Autodesk Inventor part; units mm, degrees
ref_plane "YZ Plane" through (0, 0, 0) normal (1, 0, 0) x (0, 1, 0)
ref_plane "XZ Plane" through (0, 0, 0) normal (0, 1, 0) x (-1, 0, 0)
ref_plane "XY Plane" through (0, 0, 0) normal (0, 0, 1) x (1, 0, 0)
sketch "Sketch1" plane through (0, 0, 0) normal (0, 0, 1) x (1, 0, 0)
  line L0 (0, 0) -> (177.8, 0)
  line L1 (177.8, 0) -> (177.8, 50.8)
  line L2 (177.8, 50.8) -> (0, 50.8)
  line L3 (0, 50.8) -> (0, 0)
  dimension "d0" = 177.8
  dimension "d1" = 50.8
extrude "Extrusion1" add sketch "Sketch1" along normal blind 25.4
shell "Shell1" thickness 1.5875 removed faces 2 at (0, 33.8667, 16.9333) at (177.8, 16.9333, 16.9333)
sketch "Sketch2" plane through (0, 0, 25.4) normal (0, 0, 1) x (1, 0, 0)
  line L0 (0, 0) -> (63.5, 0) construction
  line L1 (63.5, 0) -> (63.5, 25.4) construction
  line L2 (63.5, 25.4) -> (0, 25.4) construction
  line L3 (0, 25.4) -> (0, 0) construction
  dimension "d5" = 63.5
  dimension "d13" = 25.4
hole "Hole1" at (63.5, 25.4, 25.4) direction (0, 0, -1) diameter 28.575 end through all
hole "Hole2" at (12.7, 12.7, 25.4) direction (0, 0, -1) diameter 5.1594 end through all
hole "Hole3" at (38.1, 12.7, 25.4) direction (0, 0, -1) diameter 5.1594 end through all
hole "Hole4" at (165.1, 12.7, 25.4) direction (0, 0, -1) diameter 5.1594 end through all
hole "Hole5" at (139.7, 12.7, 25.4) direction (0, 0, -1) diameter 5.1594 end through all
hole "Hole6" at (12.7, 0, 12.7) direction (0, 1, 0) diameter 5.1594 depth 1.5875 tip angle 118
hole "Hole7" at (165.1, 0, 12.7) direction (0, 1, 0) diameter 5.1594 depth 3.175 tip angle 118
properties part number "1x2 5 in Beam Flywheel Mount"
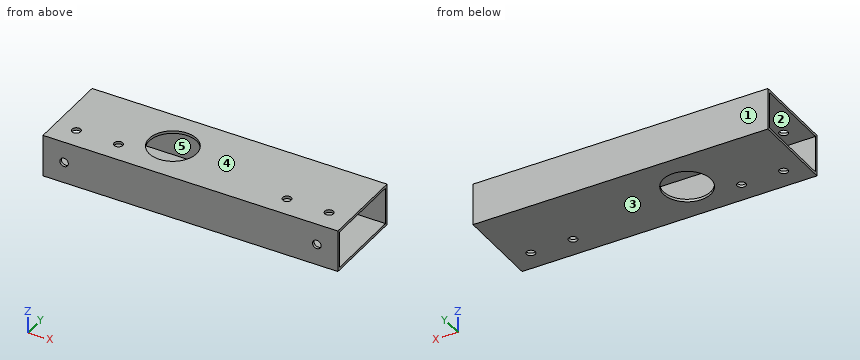
Design review of the part built by this model. Coordinates are the model's own, in mm. Face numbers are marked on the shaded views. A direction names the side the tool comes from. Round coordinates to 2 decimals unless told otherwise and drop trailing zeros. Write each loop counter-clockwise with the first axis right and the second up, starting at its lowest first coordinate (ties: lowest second). Pieces come first, ordered by that corner, then holes. Notation, with made-up numbers: (45, -18) - (97, -18) arc R11 ccw to (97, 2) - close; hole circle Ø4 at (1.25, 59). An arc over 180 degrees is marked (long way). Return JSON: item names as keys, results as strings. Group by question number.
Item 1: We need section A-A on z = 12.7. Write out the cut boundary in (x, y), and give its area (3 significant figures).
Item 2: For probe 1 along X at (y, z) = (0.6, 12.7); probe 2 along Z at (x, y) = (23.5, 4); probe 3 along Y at (x, z) = (165.1, 24.7), list the stretches that pass through material, from the lowest coordinate up. Write a range as [from, to].
Item 3: The part is to be moulded in two halves that separate along Y. For the marked faces 1, 2 and 3, say which applies: pulls with the +Y half, pulls with the -Y half, needs draft (parallel to the pull), parting line crosses it, or undercut.
Item 4: We need section D-D on x = 12.7. Write out the cut boundary in (y, z).
Item 5: We need section C-C on y = 5. Write out the cut boundary in (x, z).
Item 6: Machinability: for the marked faces 4 and 5, which of the approach directions +Z, -Z, +X, -X, +Y, -Y give a long, thin tool a straight path to every point of the face, cutting with its end or side? Answer none if there is none.
Item 7: We need section B-B on x = 38.1. Write out the cut boundary in (y, z).
Item 8: Insertion check: P1, Ø3, axis at x = 165.1, z = 12.7, coming from the -Y side; P2, Ø8.5, axis at x = 139.7, y = 12.7, coming from the -Z side. Each pin has a flat end and moves straight along its axis. Give the tip position at first contact, or say it passes through.
Model answer:
{
 "1": {"outline": "(0, 0) - (10.12, 0) - (10.12, 1.59) - (0, 1.59) - close; (0, 49.21) - (177.8, 49.21) - (177.8, 50.8) - (0, 50.8) - close; (15.28, 0) - (162.52, 0) - (162.52, 1.59) - (15.28, 1.59) - close; (167.68, 0) - (177.8, 0) - (177.8, 1.59) - (167.68, 1.59) - close", "area": "548 mm²"},
 "2": {"probe 1": "x = [0, 10.12], [15.28, 162.52], [167.68, 177.8]", "probe 2": "z = [0, 1.59], [23.81, 25.4]", "probe 3": "y = [0, 10.12], [15.28, 50.8]"},
 "3": {"face 1": "pulls with the +Y half", "face 2": "undercut", "face 3": "needs draft"},
 "4": {"outline": "(0, 0) - (10.12, 0) - (10.12, 1.59) - (1.59, 1.59) - (1.59, 10.12) - (0, 10.12) - close; (0, 15.28) - (1.59, 15.28) - (1.59, 23.81) - (10.12, 23.81) - (10.12, 25.4) - (0, 25.4) - close; (15.28, 0) - (50.8, 0) - (50.8, 25.4) - (15.28, 25.4) - (15.28, 23.81) - (49.21, 23.81) - (49.21, 1.59) - (15.28, 1.59) - close"},
 "5": {"outline": "(0, 0) - (177.8, 0) - (177.8, 1.59) - (0, 1.59) - close; (0, 23.81) - (177.8, 23.81) - (177.8, 25.4) - (0, 25.4) - close"},
 "6": {"face 4": "+Z, +X, -X, +Y, -Y", "face 5": "+X, -X"},
 "7": {"outline": "(0, 0) - (10.12, 0) - (10.12, 1.59) - (1.59, 1.59) - (1.59, 23.81) - (10.12, 23.81) - (10.12, 25.4) - (0, 25.4) - close; (15.28, 0) - (50.8, 0) - (50.8, 25.4) - (15.28, 25.4) - (15.28, 23.81) - (49.21, 23.81) - (49.21, 1.59) - (15.28, 1.59) - close"},
 "8": {"P1": "stops at y = 49.21", "P2": "stops at z = 0"}
}
